```python
from build123d import *

# Parameters (mm, degrees)
F0_R     = 10
F1_DEPTH = 10


with BuildPart() as f1:
    # F0 (on Front) → F1 (new body, symmetric)
    with BuildSketch(Plane.XZ):
        with BuildLine():
            Line((15, -250), (15, 0))
            ThreePointArc((15, 0), (0, 15), (-15, 0))
            Line((-15, 0), (-15, -250))
            ThreePointArc((-15, -250), (0, -265), (15, -250))
        make_face()
        with Locations((0, -250)):
            Circle(F0_R, mode=Mode.SUBTRACT)
        Circle(F0_R, mode=Mode.SUBTRACT)
    extrude(amount=F1_DEPTH, both=True)


solid = f1.part
```
Input: part model. Units: mm. Frame: model coordinates. Coordinates: 2 decimals unless noted, no trailing zeros. Loops run counter-clockwise (first coordinate to the right, second up) from the corner with the lowest first, then second, coordinate; pieces in that order, holes last.
Q1. Section A-A, the plane x = 0. Return the cut outline in (y, z), and give its area (3 significant figures).
Results are:
outline: (-10, -265) - (10, -265) - (10, -260) - (-10, -260) - close; (-10, -240) - (10, -240) - (10, -10) - (-10, -10) - close; (-10, 10) - (10, 10) - (10, 15) - (-10, 15) - close
area: 4,800 mm2
Q2. Section B-B, the plane z = -3.5. Return the cut outline in (x, y), and give its area (3 significant figures).
Results are:
outline: (-15, -10) - (-9.37, -10) - (-9.37, 10) - (-15, 10) - close; (9.37, -10) - (15, -10) - (15, 10) - (9.37, 10) - close
area: 225 mm2
Q3. Contact query for flat-ended pins moving along their axis: pin 1 (2 mm diameter, centred on x = -3.5, y = 1, fed in from +Z); pin 2 (1 mm diameter, centred on x = 11, y = -1.5, fed in from -Z). Output: stop coordinate, or through.
Results are:
pin 1: stops at z = 14.79
pin 2: stops at z = -260.71
Q4. Mould query, pull axis Z, two halves, no side actions, for faces 1 (the flat face through (0, -10, -123)), 2 (the cylindrical face through (-2.17, 0.14, -9.76)), 3 (the cylindrical face through (0, 0, -265)). Classes: +Z half, -Z half, draft (parallel to the pull), parting line (faces both ways), or undercut.
Results are:
face 1: draft
face 2: undercut
face 3: -Z half
Q5. Section C-C, the plane y = 5.25. Return the cut outline in (x, z), and give its area (3 significant figures).
Results are:
outline: (-15, -250) arc R15 ccw to (15, -250) - (15, 0) arc R15 ccw to (-15, 0) - close; hole circle Ø20 at (0, -250); hole circle Ø20 at (0, 0)
area: 7,580 mm2
Q6. Line query: line 1 along Z through (x, y) = (0, -5.5); line 2 along X through (y, z) = (-4.25, -249.5); line 3 along Z through (x, y) = (-5.5, 5.75). Output: solid intervals per line, ascending.
Results are:
line 1: z = -265 to -260, -240 to -10, 10 to 15
line 2: x = -15 to -9.99, 9.99 to 15
line 3: z = -263.96 to -258.35, -241.65 to -8.35, 8.35 to 13.96
